Input: part model. Units: mm. Frame: model coordinates. A direction names the side the tool comes from. Give positions to 0.01 mm unless a question says otherwise; leave off trailing zeros. Loops run counter-clockwise (first coordinate to the right, second up) from the corner with the lowest first, then second, coordinate; pieces in that order, holes last. Notation, with made-up numbers: M 81,9 L 127,9 A37 ccw 127,46 Z; hole C 56,48 d8. An arc over 180 degrees is marked long. Answer as a JSON object with one key per item and string values. Group by question number.
```python
from build123d import *

# Parameters (mm, degrees)
F2_R     = 30
F2_R_2   = 28.5
F3_DEPTH = 5
F4_R     = 1


with BuildPart() as f1:
    # F0 (on Front) → F1 (revolve)
    with BuildSketch(Plane.XZ):
        Polygon((0, 4), (0, 0), (35, 0), (35, 3), (30, 4.339746), (30, 32.57956), (26, 32.57956), (26, 4), align=None)
    revolve(axis=Axis((0, 0, 16.28978), (0, 0, 1)))

    # F2 (on face) → F3 (cut)
    with BuildSketch(Plane.XY.offset(32.57956)):
        Circle(F2_R)
        Circle(F2_R_2, mode=Mode.SUBTRACT)
    extrude(amount=-F3_DEPTH, mode=Mode.SUBTRACT)

    # F4
    f4_edges = [f1.edges().sort_by_distance(p)[0] for p in [
        (-30, 0, 4.339746),
    ]]
    fillet(f4_edges, radius=F4_R)


solid = f1.part
```
1. Section B-B (z = 21). Output: boundary loops of the cut face in (x, y).
2. Material intervals for L1, parallel to Y at x = 0, z = 24; L2, parallel to Z at x = -9, y = 2; L3, parallel to Y at x = -4.5, z = 21.5, sorted ascending.
3. Reachability of faces 1 (the flat face through (0, 0, 4)), 2 (the flat face through (0, 0, 0)) from +Z, -Z, +X, -X, +Y, -Y: full face, straight path, thin tool, end or side. Return the list, or none.
4. Mould query, pull axis X, two halves, no side actions, for faces 3 (the cylindrical face through (-20.633, -15.821, 18.09)), 4 (the cylindrical face through (-28, -21, 2)), 5 (the flat face through (23, -13, 32.58)). Classes: pulls with the +X half, pulls with the -X half, needs draft (parallel to the pull), parting line crosses it, or undercut.
5. First-contact query: P1, Ø10, axis at y = 18, z = 10.5, coming from the -X side; P2, Ø4, axis at x = -23, z = 15.5, coming from the -Y side; P3, Ø6, axis at y = -1, z = 18.5, coming from the +X side. Flat tips, straight axial feed; report the tip coordinate or a pass-through.
6. Section A-A (z = 29.5). Output: boundary loops of the cut face in (x, y).
Geometry results:
{
 "1": {"outline": "C 0,0 d60; hole C 0,0 d52"},
 "2": {"L1": "-30 to -26, 26 to 30", "L2": "0 to 4", "L3": "-29.66 to -25.61, 25.61 to 29.66"},
 "3": {"face 1": "+Z", "face 2": "-Z, +X, -X, +Y, -Y"},
 "4": {"face 3": "undercut", "face 4": "parting line crosses it", "face 5": "needs draft"},
 "5": {"P1": "x = -27.04", "P2": "y = -21.42", "P3": "x = 30"},
 "6": {"outline": "C 0,0 d57; hole C 0,0 d52"}
}
